Read the model definition and answer for the solid it produces. Units are mm, in the model's axes. Face numbers are marked on the shaded views. A direction names the side the tool comes from. Coordinates: 2 decimals unless noted, no trailing zeros. Loops run counter-clockwise (first coordinate to the right, second up) from the corner with the lowest first, then second, coordinate; pieces in that order, holes last. Notation, with made-up numbers: M -8,43 L 17,43 A33 ccw 17,75 Z; hole C 14.25,-35.5 d11. An arc over 180 degrees is marked long. One line per item, written item: value. Start each with the question number.
```python
from build123d import *

# Parameters (mm, degrees)
BOSS_EXTRUDE1_DEPTH = 50.8
SKETCH2_R           = 50.8
BOSS_EXTRUDE2_DEPTH = 19.05
SKETCH3_R           = 31.75
CUT_EXTRUDE1_DEPTH  = 102.6
CUT_EXTRUDE2_DEPTH  = 331.2
FILLET1_R           = 12.7


with BuildPart() as part:
    # Sketch1 → Boss-Extrude1 (new body, symmetric)
    with BuildSketch(Plane.XY):
        with BuildLine():
            Line((-50.8, 0), (50.8, 0))
            Line((50.8, 0), (148.497855998, 53.036837313))
            ThreePointArc((148.497855998, 53.036837313), (160.635590775, 64.705829567), (165.1, 80.940330977))
            Line((165.1, 80.940330977), (165.1, 180.036837313))
            Line((165.1, 180.036837313), (127, 180.036837313))
            Line((127, 180.036837313), (127, 82.55))
            Line((127, 82.55), (-127, 82.55))
            Line((-127, 82.55), (-127, 180.036837313))
            Line((-127, 180.036837313), (-165.1, 180.036837313))
            Line((-165.1, 180.036837313), (-165.1, 80.940330977))
            ThreePointArc((-165.1, 80.940330977), (-160.635590775, 64.705829567), (-148.497855998, 53.036837313))
            Line((-148.497855998, 53.036837313), (-50.8, 0))
        make_face()
    extrude(amount=BOSS_EXTRUDE1_DEPTH, both=True)

    # Sketch2 → Boss-Extrude2 (add)
    with BuildSketch(Plane.XZ):
        Circle(SKETCH2_R)
    extrude(amount=BOSS_EXTRUDE2_DEPTH)

    # Sketch3 → Cut-Extrude1 (cut, through all)
    with BuildSketch(Plane(origin=(0, 82.55, 0), x_dir=(1, 0, 0), z_dir=(0, 1, 0))):
        Circle(SKETCH3_R)
    extrude(amount=-CUT_EXTRUDE1_DEPTH, mode=Mode.SUBTRACT)

    # Sketch4 → Cut-Extrude2 (cut, through all)
    with BuildSketch(Plane(origin=(165.1, 0, 0), x_dir=(0, 0, -1), z_dir=(1, 0, 0))):
        Polygon((-50.8, 180.036837313), (-50.8, 80.940330977), (-38.1, 180.036837313), align=None)
        with BuildLine():
            Line((19.05, 180.036837313), (-19.05, 180.036837313))
            Line((-19.05, 180.036837313), (-19.05, 154.636837313))
            ThreePointArc((-19.05, 154.636837313), (0, 135.586837313), (19.05, 154.636837313))
            Line((19.05, 154.636837313), (19.05, 180.036837313))
        make_face()
        Polygon((38.1, 180.036837313), (50.8, 80.940330977), (50.8, 180.036837313), align=None)
    extrude(amount=-CUT_EXTRUDE2_DEPTH, mode=Mode.SUBTRACT)

    # Fillet1
    fillet1_edges = [part.edges().sort_by_distance(p)[0] for p in [
        (146.05, 180.036837313, -38.1),
        (-146.05, 180.036837313, -38.1),
        (146.05, 180.036837313, 38.1),
        (-146.05, 180.036837313, 38.1),
    ]]
    fillet(fillet1_edges, radius=FILLET1_R)


solid = part.part
```
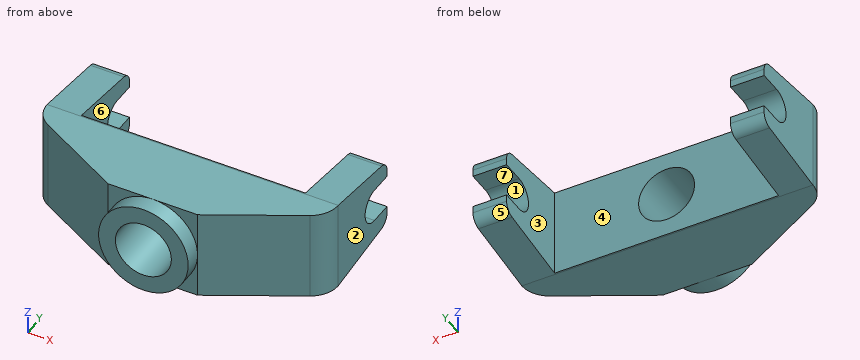
1) Section C-C (z = 43) is taken. Determine the outline of the cut face in (x, y), then the cut area to 3 significant figures.
2) For a pull along X with two mould halves and no side action, classify the marked faces 1, 2, 3 and 4 as released by +X, released by -X, zero draft, split by the parting line, or undercut.
3) A tool of negligible diameter and unlimited length cuts with its end or side. For the marked faces 5, 6 and 7, from which of +Z, -Z, +X, -X, +Y, -Y can it reach the whole face along a straight path? Write none if from no direction.
4) Consider line 1 along X through (y, z) = (103, -27); line 2 along Z through (x, y) = (0, 4); line 3 along Y through (x, z) = (-36, 39). Determine where each line is inside the solid, lowest interval first.
5) Section D-D (y = 58) is taken. Determine the outline of the cut face in (x, z), then the cut area to 3 significant figures.
6) Section A-A (y = 147.5) is taken. Determine the outline of the cut face in (x, z).
7) Section B-B (x = 13.5) is taken. Determine the outline of the cut face in (y, z), then the cut area to 3 significant figures.
8) Flat-ended cylindrical pins translate along their axes: pin 1 (2 mm diameter, centred on x = -114.5, z = 22.5, fed in from +Y); pin 2 (6 mm diameter, centred on y = 47.5, z = -24, fed in from -X); pin 3 (12.5 mm diameter, centred on x = -144, y = 169.5, fed in from +Z). Find the tip coordinate at first contact, or state that the pin passes through.
Results found:
1. outline: M -165.1,80.94 A31.75 ccw -148.5,53.04 L -50.8,0 L -27.05,0 L -27.05,-19.05 L 27.05,-19.05 L 27.05,0 L 50.8,0 L 148.5,53.04 A31.75 ccw 165.1,80.94 L 165.1,141.8 L 127,141.8 L 127,82.55 L -127,82.55 L -127,141.8 L -165.1,141.8 Z
1. area: 25,600 mm²
2. face 1: zero draft
2. face 2: released by +X
2. face 3: undercut
2. face 4: undercut
3. face 5: -Z, +X, -X, +Y
3. face 6: +Z, -Z, +Y
3. face 7: +X, -X, +Y
4. line 1: x = -165.1 to -127, 127 to 165.1
4. line 2: z = -50.8 to -31.75, 31.75 to 50.8
4. line 3: y = 0 to 82.55
5. outline: M -155.3,-50.8 L 155.3,-50.8 L 155.3,50.8 L -155.3,50.8 Z; hole C 0,0 d63.5
5. area: 28,400 mm²
6. outline: M -165.1,-42.27 L -127,-42.27 L -127,-17.66 L -165.1,-17.66 Z; M -165.1,17.66 L -127,17.66 L -127,42.27 L -165.1,42.27 Z; M 127,-42.27 L 165.1,-42.27 L 165.1,-17.66 L 127,-17.66 Z; M 127,17.66 L 165.1,17.66 L 165.1,42.27 L 127,42.27 Z
7. outline: M -19.05,-48.97 L 0,-48.97 L 0,-50.8 L 80.94,-50.8 L 82.55,-50.59 L 82.55,-28.74 L -19.05,-28.74 Z; M -19.05,28.74 L 82.55,28.74 L 82.55,50.59 L 80.94,50.8 L 0,50.8 L 0,48.97 L -19.05,48.97 Z
7. area: 4,410 mm²
8. pin 1: stops at y = 82.55
8. pin 2: stops at x = -143.82
8. pin 3: stops at z = 40.25
